Build history of the part. All positions in model axes, mm. Round coordinates to 2 decimals unless told otherwise and drop trailing zeros. Write each loop counter-clockwise with the first axis right and the second up, starting at its lowest first coordinate (ties: lowest second). Pieces come first, ordered by that corner, then holes. Notation, with made-up numbers: (-2.5, -40) -> (41.5, -40) arc R17 ccw to (41.5, -18) -> close; hole circle Ø9 at (35, 74.25). An arc over 180 degrees is marked (long way). One line per question, with ' | ' between items.
from build123d import *

# Parameters (mm, degrees)
EXTRUDE_1_DEPTH     = 0.24
CUT_EXTRUDE_1_DEPTH = 49.415468603


with BuildPart() as part:
    # 草圖1 → 填料-伸長1 (new body)
    with BuildSketch(Plane.XY):
        Polygon((8, 30), (-8, 30), (-8, 20), (-38, 20), (-38, -20), (-8, -20), (-8, -30), (8, -30), (8, -20), (38, -20), (38, 20), (8, 20), align=None)
        with BuildLine():
            Line((-0.75, -25), (-0.75, 25))
            ThreePointArc((-0.75, 25), (0, 25.75), (0.75, 25))
            Line((0.75, 25), (0.75, -25))
            ThreePointArc((0.75, -25), (0, -25.75), (-0.75, -25))
        make_face(mode=Mode.SUBTRACT)
    extrude(amount=EXTRUDE_1_DEPTH)

    # 草圖2 → 除料-伸長1 (cut, through all)
    with BuildSketch(Plane.XY.offset(0.24)):
        with BuildLine():
            Line((-8, 20), (-38, 20))
            Line((-38, 20), (-38, -20))
            Line((-38, -20), (-8, -20))
            Line((-8, -20), (-8, -19.4))
            Line((-8, -19.4), (-29.9, -19.4))
            ThreePointArc((-29.9, -19.4), (-33.435533906, -17.935533906), (-34.9, -14.4))
            Line((-34.9, -14.4), (-34.9, 14.4))
            ThreePointArc((-34.9, 14.4), (-33.435533906, 17.935533906), (-29.9, 19.4))
            Line((-29.9, 19.4), (-8, 19.4))
            Line((-8, 19.4), (-8, 20))
        make_face()
        with BuildLine():
            Line((8, 19.4), (8, 20))
            Line((8, 20), (38, 20))
            Line((38, 20), (38, -20))
            Line((38, -20), (8, -20))
            Line((8, -20), (8, -19.4))
            Line((8, -19.4), (29.9, -19.4))
            ThreePointArc((29.9, -19.4), (33.435533906, -17.935533906), (34.9, -14.4))
            Line((34.9, -14.4), (34.9, 14.4))
            ThreePointArc((34.9, 14.4), (33.435533906, 17.935533906), (29.9, 19.4))
            Line((29.9, 19.4), (8, 19.4))
        make_face()
    extrude(amount=-CUT_EXTRUDE_1_DEPTH, mode=Mode.SUBTRACT)


solid = part.part
(1) Slice it at B-B (x = 0). Write the cut outline in (y, z), then the cut area to 3 significant figures.
Calculated:
outline: (-30, 0) -> (-25.75, 0) -> (-25.75, 0.24) -> (-30, 0.24) -> close; (25.75, 0) -> (30, 0) -> (30, 0.24) -> (25.75, 0.24) -> close | area: 2.04 mm2
(2) Wall check: line 1 (X direction, y = -2, z = 0.15); line 2 (X direction, y = -22, z = 0.15); line 3 (Y direction, x = 21, z = 0.1). Give the ranges that are in metal, low to high. Write a range as from..to.
Calculated:
line 1: -34.9..-0.75, 0.75..34.9 | line 2: -8..-0.75, 0.75..8 | line 3: -19.4..19.4
(3) Slice it at D-D (x = -18). Write the cut outline in (y, z).
Calculated:
outline: (-19.4, 0) -> (19.4, 0) -> (19.4, 0.24) -> (-19.4, 0.24) -> close
(4) Slice it at C-C (z = 0.15). Write the cut outline in (x, y), then the cut area to 3 significant figures.
Calculated:
outline: (-34.9, -14.4) arc R5 ccw to (-29.9, -19.4) -> (-8, -19.4) -> (-8, -30) -> (8, -30) -> (8, -19.4) -> (29.9, -19.4) arc R5 ccw to (34.9, -14.4) -> (34.9, 14.4) arc R5 ccw to (29.9, 19.4) -> (8, 19.4) -> (8, 30) -> (-8, 30) -> (-8, 19.4) -> (-29.9, 19.4) arc R5 ccw to (-34.9, 14.4) -> close; hole (-0.75, -25) arc R0.75 ccw to (0.75, -25) -> (0.75, 25) arc R0.75 ccw to (-0.75, 25) -> close | area: 2,950 mm2
(5) Slice it at A-A (y = -5.5). Write the cut outline in (x, z), then the cut area to 3 significant figures.
Calculated:
outline: (-34.9, 0) -> (-0.75, 0) -> (-0.75, 0.24) -> (-34.9, 0.24) -> close; (0.75, 0) -> (34.9, 0) -> (34.9, 0.24) -> (0.75, 0.24) -> close | area: 16.4 mm2
